Check sheet for the drawn part. Datum: minimum x, y, z corner. Units: mm. Give positions to 0.01 mm unless a question says otherwise; leave off trailing zeros. Loops run counter-clockwise (first coordinate to the right, second up) from the corner with the lowest first, then second, coordinate; pieces in that order, holes last. Notation, with made-up numbers: (-39, 47.25) - (12, 47.25) arc R14 ccw to (12, 73.25) - close; hole circle Ø7 at (-33, 60). An arc over 180 degrees is marked (long way). Use one line per item in the form item = value.
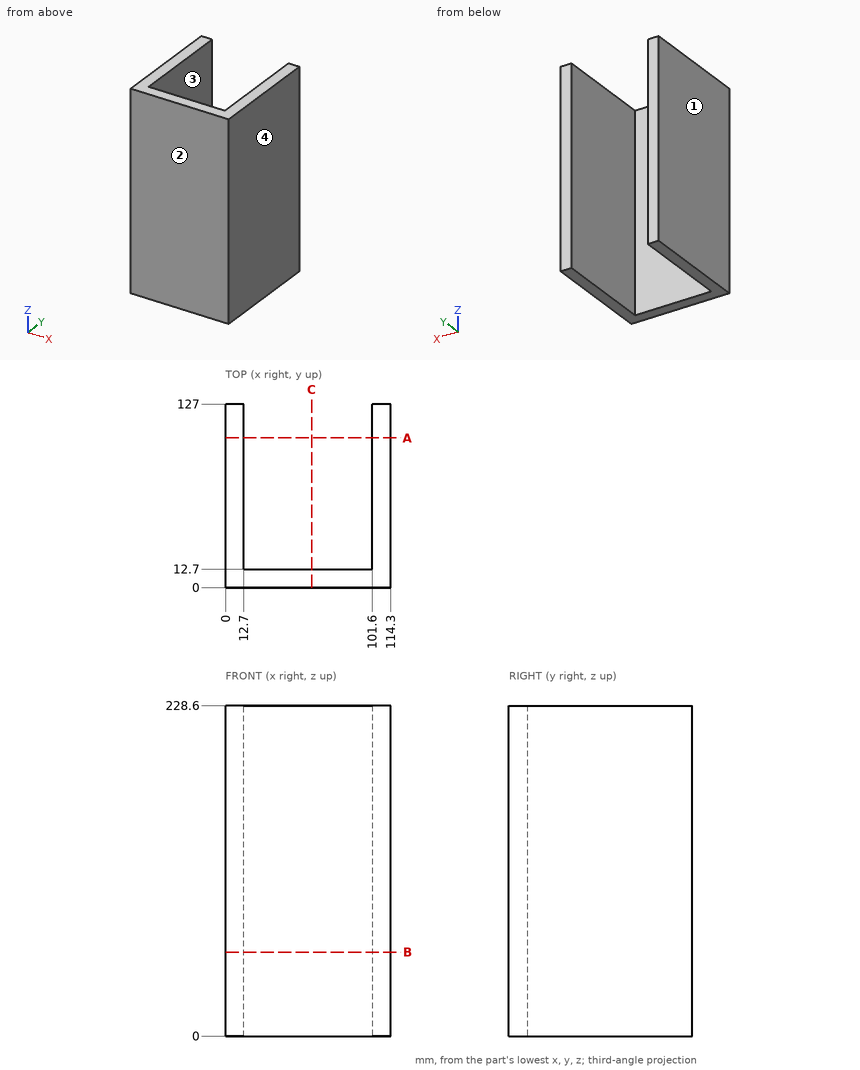
1. Section check B-B, the plane z = 58. Record the cut outline in (x, y).
Result set:
outline = (0, 0) - (114.3, 0) - (114.3, 127) - (101.6, 127) - (101.6, 12.7) - (12.7, 12.7) - (12.7, 127) - (0, 127) - close
2. Section check A-A, the plane y = 103.5. Record the cut outline in (x, z).
Result set:
outline = (0, 0) - (12.7, 0) - (12.7, 228.6) - (0, 228.6) - close; (101.6, 0) - (114.3, 0) - (114.3, 228.6) - (101.6, 228.6) - close
3. Section check C-C, the plane x = 59.5. Record the cut outline in (y, z), then the cut area to 3 significant figures.
Result set:
outline = (0, 0) - (12.7, 0) - (12.7, 228.6) - (0, 228.6) - close
area = 2,900 mm²
4. Draft check along X on the marked faces 1, 2, 3 and 4. Enter one of: released by +X, released by -X, zero draft, split by the parting line, or undercut.
Result set:
face_1 = released by -X
face_2 = zero draft
face_3 = undercut
face_4 = released by +X
5. Depth check by flat-ended pin: pin 1 Ø4 at (x, z) = (39.5, 46) entering from +Y. Enter the tip coordinate at first touch or a pass-through.
Result set:
pin_1 = 12.7
6. Scan lines: probe 1 along X at (y, z) = (82, 170.5); probe 2 along Y at (x, z) = (75.5, 68.5). Record each from-to range of solid material in increasing order.
Result set:
probe_1 = 0 to 12.7, 101.6 to 114.3
probe_2 = 0 to 12.7
